```python
from build123d import *

# Parameters (mm, degrees)
SKETCH1_W           = 174
SKETCH1_H           = 46
BOSS_EXTRUDE1_DEPTH = 18
SKETCH2_W           = 126
SKETCH2_H           = 46
CUT_EXTRUDE1_DEPTH  = 4
SKETCH3_R           = 5
CUT_EXTRUDE2_DEPTH  = 92.771455257
BOSS_EXTRUDE3_DEPTH = 14
SKETCH6_R           = 14
BOSS_EXTRUDE5_DEPTH = 2
CUT_EXTRUDE3_REACH  = 121.008
SKETCH7_R           = 7
BOSS_EXTRUDE7_DEPTH = 5
FILLET1_R           = 2
FILLET2_R           = 2


with BuildPart() as part:
    # Sketch1 → Boss-Extrude1 (new body)
    with BuildSketch(Plane.XY):
        Rectangle(SKETCH1_W, SKETCH1_H)
    extrude(amount=BOSS_EXTRUDE1_DEPTH)

    # Sketch2 → Cut-Extrude1 (cut)
    with BuildSketch(Plane(origin=(0, 0, 0), x_dir=(-1, 0, 0), z_dir=(0, 0, -1))):
        Rectangle(SKETCH2_W, SKETCH2_H)
    extrude(amount=-CUT_EXTRUDE1_DEPTH, mode=Mode.SUBTRACT)

    # Sketch3 → Cut-Extrude2 (cut, through all)
    with BuildSketch(Plane(origin=(0, 0, 0), x_dir=(-1, 0, 0), z_dir=(0, 0, -1))):
        with Locations((75, 12)):
            Circle(SKETCH3_R)
        with Locations(Location((75, -12, 0), (0, 0, 180))):
            Circle(SKETCH3_R)
        with Locations((-75, -12)):
            Circle(SKETCH3_R)
        with Locations(Location((-75, 12, 0), (0, 0, 180))):
            Circle(SKETCH3_R)
    extrude(amount=-CUT_EXTRUDE2_DEPTH, mode=Mode.SUBTRACT)

    # Sketch4 → Boss-Extrude3 (add)
    with BuildSketch(Plane.ZY.offset(32)):
        with BuildLine():
            Line((4, 23), (-32, 23))
            ThreePointArc((-32, 23), (-55, 0), (-32, -23))
            Line((-32, -23), (4, -23))
            Line((4, -23), (4, 23))
        make_face()
    boss_extrude3 = extrude(amount=-BOSS_EXTRUDE3_DEPTH)

    # Sketch6 → Boss-Extrude5 (add)
    with BuildSketch(Plane(origin=(-18, 0, 0), x_dir=(0, 0, -1), z_dir=(1, 0, 0))):
        with Locations(Location((31.952757206, 0, 0), (0, 0, 180))):
            Circle(SKETCH6_R)
    boss_extrude5 = extrude(amount=BOSS_EXTRUDE5_DEPTH)

    # Sketch7 → Cut-Extrude3 (cut, up to next)
    with BuildSketch(Plane(origin=(-16, 0, 0), x_dir=(0, 0, -1), z_dir=(1, 0, 0)), mode=Mode.PRIVATE) as cut_extrude3_sk1:
        with Locations((31.952757206, 0)):
            Circle(SKETCH7_R)
    cut_extrude3_tool1 = extrude(cut_extrude3_sk1.sketch, amount=-CUT_EXTRUDE3_REACH, mode=Mode.PRIVATE) & part.part
    cut_extrude3 = cut_extrude3_tool1.solids().sort_by_distance((-16, 0, -31.952757))[0]
    add(cut_extrude3, mode=Mode.SUBTRACT)

    # Sketch9 → Boss-Extrude7 (add, symmetric)
    with BuildSketch(Plane(origin=(0, 0, 0), x_dir=(1, 0, 0), z_dir=(0, 1, 0))):
        Polygon((-32, 20), (-63, -4), (-32, -4), align=None)
    boss_extrude7 = extrude(amount=BOSS_EXTRUDE7_DEPTH, both=True)

    # Mirror1: Boss-Extrude3, Boss-Extrude5, Cut-Extrude3, Boss-Extrude7 across plane
    add(boss_extrude3.mirror(Plane(origin=(0, 0, 0), x_dir=(0, 0, 1), z_dir=(1, 0, 0))))
    add(boss_extrude5.mirror(Plane(origin=(0, 0, 0), x_dir=(0, 0, 1), z_dir=(1, 0, 0))))
    add(cut_extrude3.mirror(Plane(origin=(0, 0, 0), x_dir=(0, 0, 1), z_dir=(1, 0, 0))), mode=Mode.SUBTRACT)
    add(boss_extrude7.mirror(Plane(origin=(0, 0, 0), x_dir=(0, 0, 1), z_dir=(1, 0, 0))))

    # Fillet1
    fillet1_edges = [part.edges().sort_by_distance(p)[0] for p in [
        (32, 14, 4),
        (-18, 0, 4),
        (-32, -14, 4),
        (-32, 14, 4),
        (32, -14, 4),
        (18, 0, 4),
    ]]
    fillet(fillet1_edges, radius=FILLET1_R)

    # Fillet2
    fillet2_edges = [part.edges().sort_by_distance(p)[0] for p in [
        (-18, 0, -45.952757206),
        (18, 0, -45.952757206),
    ]]
    fillet(fillet2_edges, radius=FILLET2_R - 0.0001)  # a hair under: the kernel refuses the full size


solid = part.part
```
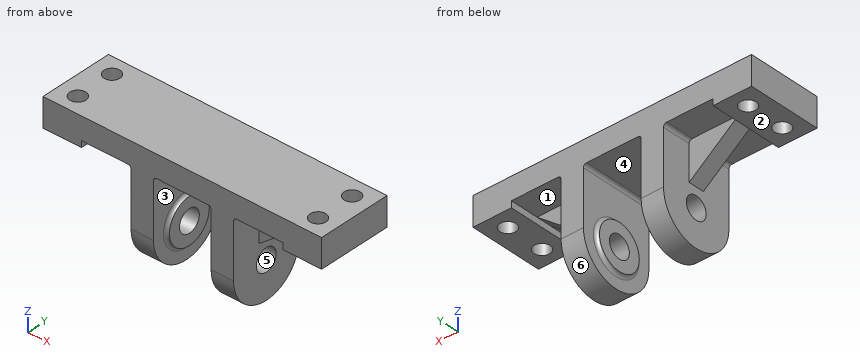
Geometry: final body of the model. Coordinates: model frame, mm. Face numbers are marked on the shaded views. A direction names the side the tool comes from. Round coordinates to 2 decimals unless told otherwise and drop trailing zeros. Write each loop counter-clockwise with the first axis right and the second up, starting at its lowest first coordinate (ties: lowest second). Pieces come first, ordered by that corner, then holes. Notation, with made-up numbers: M 43,33.25 L 79,33.25 A16 ccw 79,61.25 Z; hole C 29.5,3.5 d3. An arc over 180 degrees is marked long. Answer in a Markdown table with one row per item. Add a question column.
(1) Contact query for flat-ended pins moving along their axis: pin 1 (14 mm diameter, centred on y = 6, z = -34.5, fed in from -X); pin 2 (10 mm diameter, centred on y = -5, z = -8.5, fed in from +X); pin 3 (8 mm diameter, centred on x = -23, y = -2.5, fed in from -Z). Output: stop coordinate, or through.
(2) Cut plane A-A, the plane x = 75. Return the cut outline in (y, z), then the cut area to 3 significant figures.
(3) Cut plane B-B, the plane x = -30. Return the cut outline in (y, z).
(4) Cut plane C-C, the plane z = -4.5. Return the cut outline in (x, y).
(5) Draft query along Y for the marked faces 4, 5 and 6. Return one class per face: pulls with the +Y half, pulls with the -Y half, needs draft (parallel to the pull), parting line crosses it, or undercut.
(6) Ray query, L1, parallel to Y at x = 75, z = 7; L2, parallel to X at y = -17.5, z = -30; L3, parallel to X at y = 10.5, z = -29.5. Return the intervals inside material, ascending.
(7) Cut plane D-D, the plane x = -72. Return the cut outline in (y, z), then the cut area to 3 significant figures.
(8) Reachability of the marked faces 1, 2 and 3 from +Z, -Z, +X, -X, +Y, -Y: full face, straight path, thin tool, end or side. Return the list, or none.
Established:
| question | item | result |
|---|---|---|
| 1 | pin 1 | x = -32 |
| 1 | pin 2 | x = 53.31 |
| 1 | pin 3 | z = -55 |
| 2 | outline | M -23,0 L -17,0 L -17,18 L -23,18 Z; M -7,0 L 7,0 L 7,18 L -7,18 Z; M 17,0 L 23,0 L 23,18 L 17,18 Z |
| 2 | area | 468 mm² |
| 3 | outline | M -23,-32 A23 ccw 23,-32 L 23,18 L -23,18 Z; hole C 0,-31.95 d14 |
| 4 | outline | M -52.02,-5 L -32,-5 L -32,-23 L -18,-23 L -18,23 L -32,23 L -32,5 L -52.02,5 Z; M 18,-23 L 32,-23 L 32,-5 L 52.02,-5 L 52.02,5 L 32,5 L 32,23 L 18,23 Z |
| 5 | face 4 | needs draft |
| 5 | face 5 | undercut |
| 5 | face 6 | parting line crosses it |
| 6 | L1 | -23 to -17, -7 to 7, 17 to 23 |
| 6 | L2 | -32 to -18, 18 to 32 |
| 6 | L3 | -32 to -16, 16 to 32 |
| 7 | outline | M -23,0 L -16,0 L -16,18 L -23,18 Z; M -8,0 L 8,0 L 8,18 L -8,18 Z; M 16,0 L 23,0 L 23,18 L 16,18 Z |
| 7 | area | 540 mm² |
| 8 | face 1 | -Z, +Y |
| 8 | face 2 | -Z, -X, +Y, -Y |
| 8 | face 3 | none |
